The model under review builds one solid part; all positions refer to its coordinate system, in mm. Face numbers are marked on the shaded views. A direction names the side the tool comes from. Coordinates: 2 decimals unless noted, no trailing zeros. Order: outer loops, then holes, each group sorted by start corner. A loop starts at its lowest first (then second) coordinate and runs counter-clockwise, first axis right, second up.
```python
from build123d import *

# Parameters (mm, degrees)
CROQUIS1_W            = 2
CROQUIS1_H            = 10
CORTAR_EXTRUIR2_DEPTH = 2
CHAFL_N3_SIZE         = 0.3
CHAFL_N4_SIZE         = 0.15


with BuildPart() as part:
    # Croquis1 → Revolución1 (revolve)
    with BuildSketch(Plane.XY, mode=Mode.PRIVATE) as revoluci_n1_sk:
        with Locations((1, -5)):
            Rectangle(CROQUIS1_W, CROQUIS1_H)
    revolve(revoluci_n1_sk.sketch.rotate(Axis((0, 0, 0), (0, -1, 0)), 90), axis=Axis((0, 0, 0), (0, -1, 0)))

    # Croquis3 → Cortar-Extruir2 (cut)
    with BuildSketch(Plane(origin=(0, 0, 0), x_dir=(1, 0, 0), z_dir=(0, 1, 0))):
        Polygon((-0.577350269, 1), (-1.154700538, 0), (-0.577350269, -1), (0.577350269, -1), (1.154700538, 0), (0.577350269, 1), align=None)
    extrude(amount=-CORTAR_EXTRUIR2_DEPTH, mode=Mode.SUBTRACT)

    # Chaflán3
    chafl_n3_edges = [part.edges().sort_by_distance(p)[0] for p in [
        (0, -10, -2),
    ]]
    chamfer(chafl_n3_edges, length=CHAFL_N3_SIZE)

    # Chaflán4
    chafl_n4_edges = [part.edges().sort_by_distance(p)[0] for p in [
        (0, 0, -2),
    ]]
    chamfer(chafl_n4_edges, length=CHAFL_N4_SIZE)


solid = part.part
```
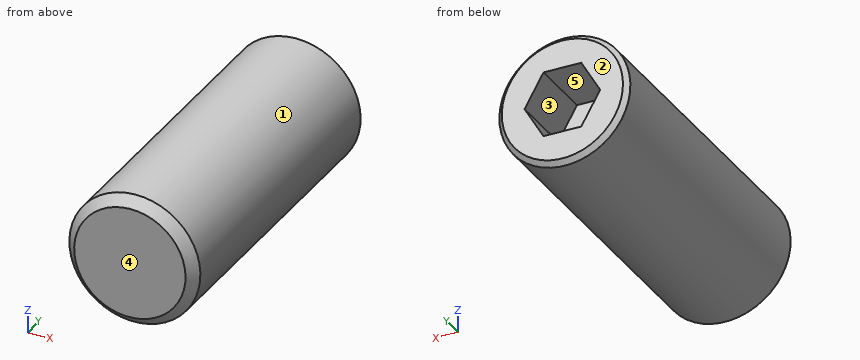
(1) Machinability: for the marked faces 4 and 5, which of the approach directions +Z, -Z, +X, -X, +Y, -Y give a long, thin tool a straight path to every point of the face, cutting with its end or side? Answer none if there is none.
A:
face 4: +Z, -Z, +X, -X, -Y
face 5: +Y
(2) We need section B-B, the plane y = -7.5. Write out the cut boundary in (x, z).
A:
outline: circle Ø4 at (0, 0)
(3) For pin 1 Ø1 at (x, z) = (-0.5, 0.5) entering from +Y, flat-tipped, find the tip position at first contact; note if it passes through.
A:
pin 1: stops at y = 0
(4) We need section A-A, the plane x = 0. Write out the cut boundary in (y, z), and give its area (3 significant figures).
A:
outline: (-10, -1.7) - (-9.7, -2) - (-0.15, -2) - (0, -1.85) - (0, -1) - (-2, -1) - (-2, 1) - (0, 1) - (0, 1.85) - (-0.15, 2) - (-9.7, 2) - (-10, 1.7) - close
area: 35.9 mm2
(5) Draft analysis for pull direction X (two halves, no side actions). For the marked faces 1, 2 and 3, state which applies: released by +X, released by -X, zero draft, split by the parting line, or undercut.
A:
face 1: split by the parting line
face 2: zero draft
face 3: undercut
(6) Wall thickness on probe 1 along Z at (x, y) = (0.05, -1.5); probe 2 along Y at (x, z) = (0.35, -0.1); probe 3 along X at (y, z) = (-1, 0.45): over which ranges is each line inside the solid? List them lowest first.
A:
probe 1: z = -2 to -1, 1 to 2
probe 2: y = -10 to -2
probe 3: x = -1.95 to -0.89, 0.89 to 1.95
